from build123d import *

# Parameters (mm, degrees)
ESQUISSE1_W                  = 188
ESQUISSE1_H                  = 81.33
BOSS_EXTRU_1_DEPTH           = 6
ENL_V_MAT_EXTRU_2_DEPTH      = 205.925764364
ENL_V_MAT_EXTRU_2_DEPTH_BACK = 205.925764364
ESQUISSE4_W                  = 6
ESQUISSE4_H                  = 31.567534009
BOSS_EXTRU_2_DEPTH           = 6
ESQUISSE5_W                  = 6
ESQUISSE5_H                  = 31.067534009
BOSS_EXTRU_3_DEPTH           = 6
ESQUISSE6_W                  = 37
ESQUISSE6_H                  = 6
ENL_V_MAT_EXTRU_3_DEPTH      = 6
ESQUISSE7_R                  = 2.995
ENL_V_MAT_EXTRU_4_DEPTH      = 3
ESQUISSE8_R                  = 1.5
ENL_V_MAT_EXTRU_5_DEPTH      = 6
ESQUISSE9_R                  = 1.2
ENL_V_MAT_EXTRU_6_DEPTH      = 10


with BuildPart() as part:
    # Esquisse1 → Boss.-Extru.1 (new body)
    with BuildSketch(Plane.XY):
        with Locations((-94, 40.665)):
            Rectangle(ESQUISSE1_W, ESQUISSE1_H)
    extrude(amount=BOSS_EXTRU_1_DEPTH)

    # Esquisse2 → Enlèv. mat.-Extru.2 (cut, two sides: drawn at the far end of the back side and taken through both)
    with BuildSketch(Plane.ZY.offset(188).offset(-ENL_V_MAT_EXTRU_2_DEPTH_BACK)):
        Polygon((178.443334928, 96.416836907), (6, 81.33), (0, 80.805068019), (-172.443334928, 65.718231112), (-202.617008742, 410.604900969), (148.269661115, 441.303506764), align=None)
    extrude(amount=ENL_V_MAT_EXTRU_2_DEPTH + ENL_V_MAT_EXTRU_2_DEPTH_BACK, mode=Mode.SUBTRACT)

    # Esquisse4 → Boss.-Extru.2 (add)
    with BuildSketch(Plane.ZY.offset(188)):
        with Locations((3, 40.283767005)):
            Rectangle(ESQUISSE4_W, ESQUISSE4_H)
    extrude(amount=BOSS_EXTRU_2_DEPTH)

    # Esquisse5 → Boss.-Extru.3 (add)
    with BuildSketch(Plane(origin=(0, 0, 0), x_dir=(0, 0, -1), z_dir=(1, 0, 0))):
        with Locations((-3, 40.533767005)):
            Rectangle(ESQUISSE5_W, ESQUISSE5_H)
    extrude(amount=BOSS_EXTRU_3_DEPTH)

    # Esquisse6 → Enlèv. mat.-Extru.3 (cut)
    with BuildSketch(Plane.XY.offset(6)):
        with Locations((-131.5, 78.33)):
            Rectangle(ESQUISSE6_W, ESQUISSE6_H)
        with Locations((-56.5, 78.33)):
            Rectangle(ESQUISSE6_W, ESQUISSE6_H)
    extrude(amount=-ENL_V_MAT_EXTRU_3_DEPTH, mode=Mode.SUBTRACT)

    # Esquisse7 → Enlèv. mat.-Extru.4 (cut)
    with BuildSketch(Plane(origin=(0, 0, 0), x_dir=(-1, 0, 0), z_dir=(0, 0, -1))):
        with Locations((94, 77.805068019)):
            Circle(ESQUISSE7_R)
        with Locations((19, 77.805068019)):
            Circle(ESQUISSE7_R)
        with Locations((169, 77.805068019)):
            Circle(ESQUISSE7_R)
        with Locations((191, 40.567534009)):
            Circle(ESQUISSE7_R)
        with Locations((-3.034014412, 40.567534009)):
            Circle(ESQUISSE7_R)
    extrude(amount=-ENL_V_MAT_EXTRU_4_DEPTH, mode=Mode.SUBTRACT)

    # Esquisse8 → Enlèv. mat.-Extru.5 (cut)
    with BuildSketch(Plane(origin=(0, 0, 0), x_dir=(-1, 0, 0), z_dir=(0, 0, -1))):
        with Locations((-3.034014412, 40.567534009)):
            Circle(ESQUISSE8_R)
        with Locations((19, 77.805068019)):
            Circle(ESQUISSE8_R)
        with Locations((94, 77.805068019)):
            Circle(ESQUISSE8_R)
        with Locations((169, 77.805068019)):
            Circle(ESQUISSE8_R)
        with Locations((191, 40.567534009)):
            Circle(ESQUISSE8_R)
    extrude(amount=-ENL_V_MAT_EXTRU_5_DEPTH, mode=Mode.SUBTRACT)

    # Esquisse9 → Enlèv. mat.-Extru.6 (cut)
    with BuildSketch(Plane.XY.offset(6)):
        with Locations((-24, 68.33)):
            Circle(ESQUISSE9_R)
        with Locations((-24, 52.33)):
            Circle(ESQUISSE9_R)
        with Locations((-40, 68.33)):
            Circle(ESQUISSE9_R)
        with Locations((-40, 52.33)):
            Circle(ESQUISSE9_R)
    extrude(amount=-ENL_V_MAT_EXTRU_6_DEPTH, mode=Mode.SUBTRACT)


solid = part.part
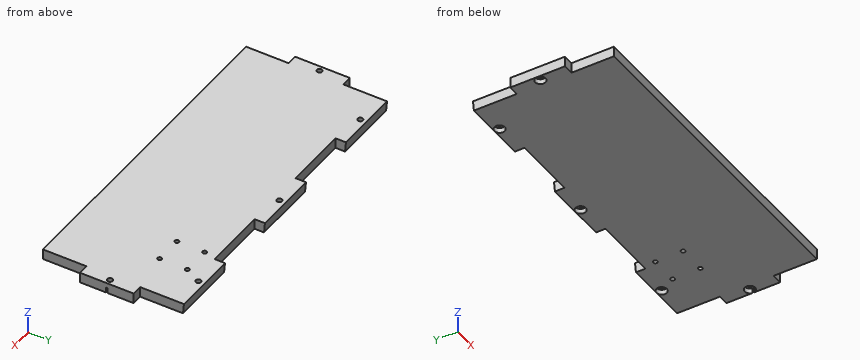
Design review of the part built by this model. Coordinates are the model's own, in mm. Give positions to 0.01 mm unless a question says otherwise; leave off trailing zeros. Write each loop counter-clockwise with the first axis right and the second up, starting at its lowest first coordinate (ties: lowest second). Pieces come first, ordered by that corner, then holes. Notation, with made-up numbers: M 49,-31 L 70,-31 A17 cw 70,-10 Z; hole C 39.5,8.5 d10. An arc over 180 degrees is marked long. Return JSON: item names as keys, results as strings. Group by question number.
Item 1: Wall thickness on line 1 along Y through (x, z) = (-24, 1.4); line 2 along X through (y, z) = (78, 4.9); line 3 along Y through (x, z) = (-191, 1.6): over which ranges is each line inside the solid? List them lowest first.
Item 2: Clearance check with flat-ended pins moving along their axes: pin 1 Ø1.8 at (x, y) = (-190, 39) entering from -Z; pin 2 Ø2.5 at (x, y) = (-191, 40.57) entering from -Z; pin 3 Ø1 at (x, z) = (-168, 4) entering from +Y; pin 4 Ø3 at (x, z) = (-55.5, 2) entering from +Y. State where each tip first meets the part, or that it passes through.
Item 3: Take a section at B-B (x = -143). Give the boundary of the cut face in (y, z), plus the area to 3 significant figures.
Item 4: Take a section at A-A (z = 4.95). Count the separate pieces of the cut face and the enclosed holes in it, plus the area to 3 significant figures.
Return value:
{
 "1": {"line 1": "y = 0 to 51.13, 53.53 to 67.13, 69.53 to 80.93", "line 2": "x = -188 to -170.49, -167.51 to -150, -113 to -95.49, -92.51 to -75, -38 to -20.49, -17.51 to 0", "line 3": "y = 24.5 to 37.57, 43.56 to 56.07"},
 "2": {"pin 1": "stops at z = 3", "pin 2": "passes through", "pin 3": "stops at y = 81.2", "pin 4": "stops at y = 75.33"},
 "3": {"outline": "M 0,0 L 75.33,0 L 75.33,6 L 0,6 Z", "area": "452 mm2"},
 "4": {"separate pieces": "1", "enclosed holes": "9", "area": "15,200 mm2"}
}
